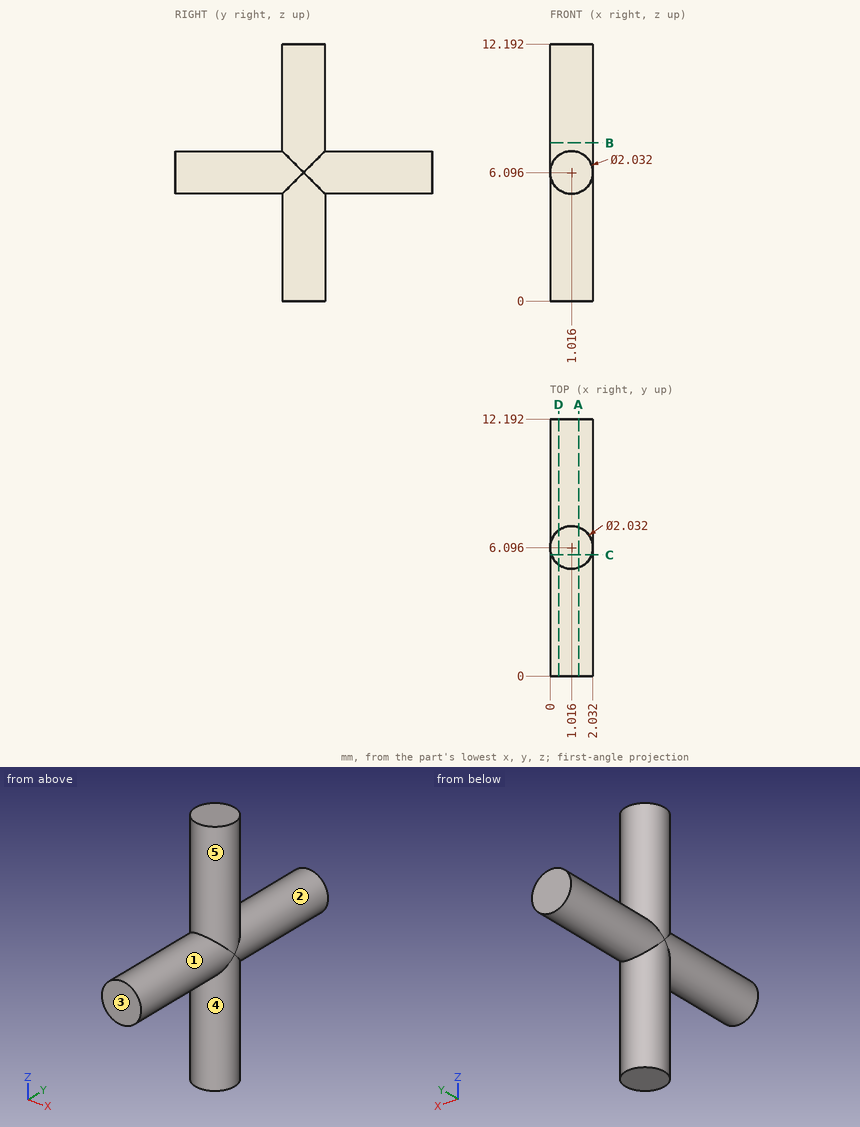
Geometry: see drawing. Coordinates: mm, zero at the bounding-box minimum. A direction names the side the tool comes from. Give positions to 0.01 mm unless a question says otherwise; leave off trailing zeros. Order: outer loops, then holes, each group sorted by start corner. A loop starts at its lowest first (then second) coordinate and runs counter-clockwise, first axis right, second up. Notation, with made-up numbers: (56, -10) - (65, -10) arc R14 cw to (65, -6) - close; hole circle Ø1 at (-22.75, 83). An arc over 180 degrees is marked (long way). Use a Markdown table: item, result.
(1) Access query for the marked faces 1, 2, 3, 4 and 5. Directions: +Z, -Z, +X, -X, +Y, -Y. A direction counts if a zero-diameter tool reaches every point of the face in a straight line with its end or side. Return the directions, or none.
Computed values:
| item | result |
|---|---|
| face 1 | -Y |
| face 2 | +Y |
| face 3 | +Z, -Z, +X, -X, -Y |
| face 4 | -Z |
| face 5 | +Z |
(2) Section query A-A (x = 1.35). Output: boundary loops of the cut face in (y, z), then the cut area to 3 significant figures.
Computed values:
| item | result |
|---|---|
| outline | (0, 5.14) - (5.14, 5.14) - (5.14, 0) - (7.06, 0) - (7.06, 5.14) - (12.19, 5.14) - (12.19, 7.06) - (7.06, 7.06) - (7.06, 12.19) - (5.14, 12.19) - (5.14, 7.06) - (0, 7.06) - close |
| area | 43.1 mm2 |
(3) Section query D-D (x = 0.4). Output: boundary loops of the cut face in (y, z), then the cut area to 3 significant figures.
Computed values:
| item | result |
|---|---|
| outline | (0, 5.29) - (5.29, 5.29) - (5.29, 0) - (6.9, 0) - (6.9, 5.29) - (12.19, 5.29) - (12.19, 6.9) - (6.9, 6.9) - (6.9, 12.19) - (5.29, 12.19) - (5.29, 6.9) - (0, 6.9) - close |
| area | 36.8 mm2 |
(4) Section query C-C (y = 5.75). Output: boundary loops of the cut face in (x, z).
Computed values:
| item | result |
|---|---|
| outline | (0.06, 0) - (1.97, 0) - (1.97, 5.75) arc R1.02 ccw to (1.97, 6.44) - (1.97, 12.19) - (0.06, 12.19) - (0.06, 6.44) arc R1.02 ccw to (0.06, 5.75) - close |
(5) Pin query (flat end, axial travel): pin 1 (1 mm diameter, centred on y = 6.5, z = 8, fed in from +X); pin 2 (2 mm diameter, centred on y = 4, z = 10.5, fed in from +X); pin 3 (6 mm diameter, centred on y = 9.5, z = 9.5, fed in from -X). Return the tip coordinate at first contact, or that it passes through.
Computed values:
| item | result |
|---|---|
| pin 1 | stops at x = 2.03 |
| pin 2 | passes through |
| pin 3 | stops at x = 0.08 |
(6) Line query: line 1 (Z direction, x = 1.1, y = 7.5); line 2 (Y direction, x = 1.2, z = 3.75); line 3 (Z direction, x = 1.7, y = 3). Output: solid intervals per line, ascending. Write a range as from..to.
Computed values:
| item | result |
|---|---|
| line 1 | z = 5.08..7.11 |
| line 2 | y = 5.1..7.1 |
| line 3 | z = 5.34..6.85 |
(7) Section query B-B (z = 7.5). Output: boundary loops of the cut face in (x, y), then the cut area to 3 significant figures.
Computed values:
| item | result |
|---|---|
| outline | circle Ø2.03 at (1.02, 6.1) |
| area | 3.24 mm2 |
